Autodesk Inventor part; units mm, degrees
ref_plane "YZ Plane" through (0, 0, 0) normal (1, 0, 0) x (0, 1, 0)
ref_plane "XZ Plane" through (0, 0, 0) normal (0, 1, 0) x (-1, 0, 0)
ref_plane "XY Plane" through (0, 0, 0) normal (0, 0, 1) x (1, 0, 0)
sketch "Sketch1" plane through (0, 0, 0) normal (0, 0, 1) x (1, 0, 0)
  line L0 (0, 0) -> (41, 0)
  line L1 (41, 0) -> (41, 30)
  line L2 (41, 30) -> (0, 30)
  line L3 (0, 30) -> (0, 0)
  line L4 (29.4, 25) -> (32.5, 25)
  line L5 (32.5, 25) -> (32.5, 5)
  line L6 (32.5, 5) -> (29.4, 5)
  line L7 (29.4, 5) -> (29.4, 25)
  line L8 (8.5, 25) -> (11.6, 25)
  line L9 (11.6, 25) -> (11.6, 5)
  line L10 (11.6, 5) -> (8.5, 5)
  line L11 (8.5, 5) -> (8.5, 25)
  point P0 (8.5, 15)
  point P1 (0, 15)
  point P2 (29.4, 15)
  point P3 (10.05, 5)
  point P4 (20.5, 30)
  dimension "d0" = 41
  dimension "d1" = 30
  dimension "d2" = 3.1
  dimension "d3" = 3.1
  dimension "d4" = 24
  dimension "d6" = 10
  dimension "d7" = 8.9
extrude "Extrusion1" add sketch "Sketch1" along normal blind 3
properties part number "Moving_rail"
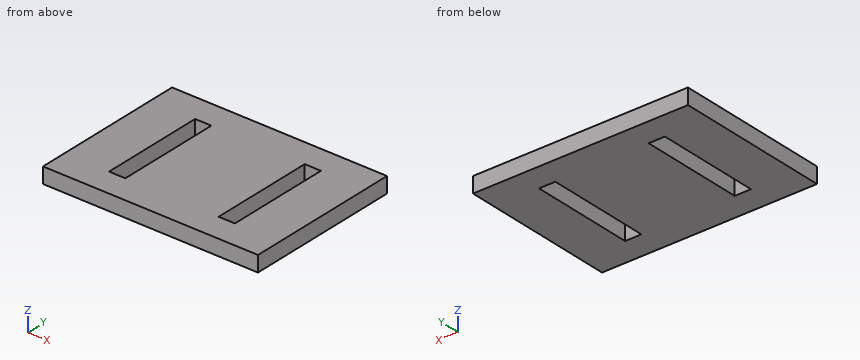
CAD build for the part. Positions are in the model's coordinates, mm. Round coordinates to 2 decimals unless told otherwise and drop trailing zeros. Write each loop counter-clockwise with the first axis right and the second up, starting at its lowest first coordinate (ties: lowest second). Pieces come first, ordered by that corner, then holes. Notation, with made-up numbers: M 29,-11.5 L 77,-11.5 A13 ccw 77,-5.5 Z; hole C -12.5,71 d8. An arc over 180 degrees is marked long. Use a Markdown table: item, result. Add a question column.
1. Slice it at A-A on y = 17. Give the cut face in (x, z).
2. Drill centre lines: probe 1 along X at (y, z) = (18.25, 0.3); probe 2 along Y at (x, z) = (9.5, 1.8). Where is each one in solid material? Low to high.
3. Slice it at B-B on z = 1.35. Give the cut face in (x, y), then the cut area to 3 significant figures.
4. Flat gauge pin, fed straight in: P1, Ø4, axis at x = 19.5, y = 10.5, coming from the -Z side. Where does the tip first touch, or does it go through?
Reply:
| question | item | result |
|---|---|---|
| 1 | outline | M 0,0 L 8.5,0 L 8.5,3 L 0,3 Z; M 11.6,0 L 29.4,0 L 29.4,3 L 11.6,3 Z; M 32.5,0 L 41,0 L 41,3 L 32.5,3 Z |
| 2 | probe 1 | x = 0 to 8.5, 11.6 to 29.4, 32.5 to 41 |
| 2 | probe 2 | y = 0 to 5, 25 to 30 |
| 3 | outline | M 0,0 L 41,0 L 41,30 L 0,30 Z; hole M 8.5,5 L 11.6,5 L 11.6,25 L 8.5,25 Z; hole M 29.4,5 L 32.5,5 L 32.5,25 L 29.4,25 Z |
| 3 | area | 1,110 mm^2 |
| 4 | P1 | stops at z = 0 |
